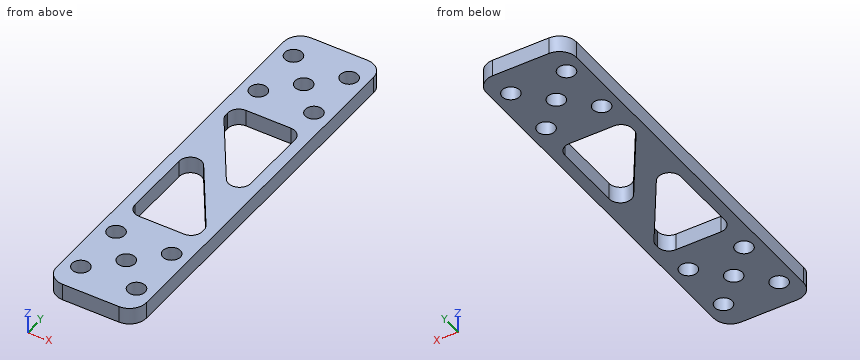
from build123d import *

# Parameters (mm, degrees)
SKETCH_1_R          = 1.55
EXTRUDE_1_DEPTH     = 3
SKETCH_2_W          = 30.67898901
SKETCH_2_H          = 20.291672983
CUT_EXTRUDE_1_DEPTH = 10
SKETCH_3_R          = 1
CUT_EXTRUDE_2_DEPTH = 20
SKETCH_4_W          = 23.960943262
SKETCH_4_H          = 52.328724607
CUT_EXTRUDE_3_DEPTH = 10
FILLET_1_R          = 3
CUT_EXTRUDE_4_DEPTH = 55.457683839
FILLET_2_R          = 2


with BuildPart() as part:
    # 草图1 → 凸台-拉伸1 (new body)
    with BuildSketch(Plane.XY):
        with BuildLine():
            Line((5, 16.216737463), (-5, 16.216737463))
            ThreePointArc((-5, 16.216737463), (-7.121320344, 15.338057806), (-8, 13.216737463))
            Line((-8, 13.216737463), (-8, -66.783262537))
            Line((-8, -66.783262537), (-4, -108.783262537))
            Line((-4, -108.783262537), (4, -108.783262537))
            Line((4, -108.783262537), (8, -66.783262537))
            Line((8, -66.783262537), (8, 13.216737463))
            ThreePointArc((8, 13.216737463), (7.121320344, 15.338057806), (5, 16.216737463))
        make_face()
        with Locations((-4.949747468, 11.166484931)):
            Circle(SKETCH_1_R, mode=Mode.SUBTRACT)
        with Locations((4.949747468, 11.166484931)):
            Circle(SKETCH_1_R, mode=Mode.SUBTRACT)
        with Locations((4.949747468, 1.266989995)):
            Circle(SKETCH_1_R, mode=Mode.SUBTRACT)
        with Locations((-4.949747468, 1.266989995)):
            Circle(SKETCH_1_R, mode=Mode.SUBTRACT)
        with Locations((0, -43.783262537)):
            Circle(SKETCH_1_R, mode=Mode.SUBTRACT)
        with Locations((4.949747468, -38.833515069)):
            Circle(SKETCH_1_R, mode=Mode.SUBTRACT)
        with Locations((-4.949747468, -38.833515069)):
            Circle(SKETCH_1_R, mode=Mode.SUBTRACT)
        with Locations((4.949747468, -48.733010005)):
            Circle(SKETCH_1_R, mode=Mode.SUBTRACT)
        with Locations((-4.949747468, -48.733010005)):
            Circle(SKETCH_1_R, mode=Mode.SUBTRACT)
        with Locations((0, 6.216737463)):
            Circle(SKETCH_1_R, mode=Mode.SUBTRACT)
    extrude(amount=EXTRUDE_1_DEPTH)

    # 草图2 → 切除-拉伸1 (cut)
    with BuildSketch(Plane(origin=(0, 0, 0), x_dir=(-1, 0, 0), z_dir=(0, 0, -1))):
        with Locations((1.230440634, -108.929099029)):
            Rectangle(SKETCH_2_W, SKETCH_2_H)
    extrude(amount=-CUT_EXTRUDE_1_DEPTH, mode=Mode.SUBTRACT)

    # 草图3 → 切除-拉伸2 (cut)
    with BuildSketch(Plane(origin=(0, 0, 0), x_dir=(-1, 0, 0), z_dir=(0, 0, -1))):
        with Locations((0, -83.783262537)):
            Circle(SKETCH_3_R)
        with Locations((0, -90.783262537)):
            Circle(SKETCH_3_R)
        with Locations((0, -73.783262537)):
            Circle(SKETCH_3_R)
    extrude(amount=-CUT_EXTRUDE_2_DEPTH, mode=Mode.SUBTRACT)

    # 草图4 → 切除-拉伸3 (cut)
    with BuildSketch(Plane(origin=(0, 0, 0), x_dir=(-1, 0, 0), z_dir=(0, 0, -1))):
        with Locations((3.980471631, -79.947624841)):
            Rectangle(SKETCH_4_W, SKETCH_4_H)
    extrude(amount=-CUT_EXTRUDE_3_DEPTH, mode=Mode.SUBTRACT)

    # 圆角1
    fillet_1_edges = [part.edges().sort_by_distance(p)[0] for p in [
        (8, -53.783262537, 1.5),
        (-8, -53.783262537, 1.5),
    ]]
    fillet(fillet_1_edges, radius=FILLET_1_R)

    # 草图5 → 切除-拉伸4 (cut, through all)
    with BuildSketch(Plane(origin=(0, 0, 0), x_dir=(-1, 0, 0), z_dir=(0, 0, -1))):
        Polygon((2, -18.783262537), (-6, -30.783262537), (-6, -33.833515069), (6, -33.833515069), (6, -18.783262537), align=None)
        Polygon((6, -3.733010005), (-6, -3.733010005), (-6, -18.783262537), (-2, -18.783262537), (6, -6.783262537), align=None)
        Polygon((-2, -18.783262537), (-6, -18.783262537), (-6, -24.783262537), align=None)
        Polygon((6, -18.783262537), (6, -12.783262537), (2, -18.783262537), align=None)
    extrude(amount=-CUT_EXTRUDE_4_DEPTH, mode=Mode.SUBTRACT)

    # 圆角2
    fillet_2_edges = [part.edges().sort_by_distance(p)[0] for p in [
        (-6, -12.783262537, 1.5),
        (-6, -33.833515069, 1.5),
        (6, -33.833515069, 1.5),
        (6, -30.783262537, 1.5),
        (6, -24.783262537, 1.5),
        (6, -3.733010005, 1.5),
        (-6, -3.733010005, 1.5),
        (-6, -6.783262537, 1.5),
    ]]
    fillet(fillet_2_edges, radius=FILLET_2_R)


solid = part.part
Could you check a few things on this model? Use its own coordinates, in mm. Give positions to 0.01 mm unless a question says otherwise; leave off trailing zeros. Loops run counter-clockwise (first coordinate to the right, second up) from the corner with the lowest first, then second, coordinate; pieces in that order, holes last. Notation, with made-up numbers: (32.25, -23) -> (91.25, -23) arc R27 cw to (91.25, -5) -> close; hole circle Ø10 at (40.25, 28). An arc over 180 degrees is marked (long way). Answer as CSV lines item,"result". Start each with the question number.
(1) If we section it at A-A on x = 0: Write out the boundary of the cut face in (y, z), then the cut area to 3 significant figures.
(2) I need wall thicknesses on probe 1 along Y at (x, z) = (-1.75, 0.4); probe 2 along X at (y, z) = (-20, 0.4); probe 3 along Y at (x, z) = (0, 1.5). Which ranges of each line are inside material? Lowest first, please.
(3) I'm going to push flat-ended pins straight in: pin 1 Ø1.9 at (x, y) = (0, 6.22) entering from -Z; pin 2 Ø3.5 at (x, y) = (4.95, -48.73) entering from -Z. Where does each tip first touch, or does it pass through?
(4) If we section it at B-B on z = 1.4: Count the separate pieces of the cut face and the enclosed holes in it, then the cut area to 3 significant figures.
Computed:
1,outline,"(-53.78, 0) -> (-45.33, 0) -> (-45.33, 3) -> (-53.78, 3) -> close; (-42.23, 0) -> (-33.83, 0) -> (-33.83, 3) -> (-42.23, 3) -> close; (-21.78, 0) -> (-15.78, 0) -> (-15.78, 3) -> (-21.78, 3) -> close; (-3.73, 0) -> (4.67, 0) -> (4.67, 3) -> (-3.73, 3) -> close; (7.77, 0) -> (16.22, 0) -> (16.22, 3) -> (7.77, 3) -> close"
1,area,"119 mm2"
2,probe 1,"y = -53.78 to -33.83, -19.16 to -13.16, -3.73 to 16.22"
2,probe 2,"x = -8 to -6, -1.19 to 3.18, 4.82 to 8"
2,probe 3,"y = -53.78 to -45.33, -42.23 to -33.83, -21.78 to -15.78, -3.73 to 4.67, 7.77 to 16.22"
3,pin 1,"passes through"
3,pin 2,"stops at z = 0"
4,separate pieces,"1"
4,enclosed holes,"12"
4,area,"767 mm2"
